Read the model definition and answer for the solid it produces. Units are mm, in the model's axes. Face numbers are marked on the shaded views. A direction names the side the tool comes from. Round coordinates to 2 decimals unless told otherwise and drop trailing zeros. Write each loop counter-clockwise with the first axis right and the second up, starting at its lowest first coordinate (ties: lowest second). Pieces come first, ordered by that corner, then holes. Notation, with made-up numbers: (-25.5, 51) -> (31.5, 51) arc R20 cw to (31.5, 77) -> close; hole circle Ø8 at (53.5, -36.75). An arc over 180 degrees is marked (long way). Return JSON: item names as keys, results as strings.
from build123d import *

# Parameters (mm, degrees)
F2_R = 0.15


with BuildPart() as f1:
    # F0 (on Front) → F1 (revolve)
    with BuildSketch(Plane.XZ):
        Polygon((-2, 2.75), (-2, 1.5), (2, 1.5), (2, 2.75), (1.5, 2.75), (1.5, 3.75), (2, 3.75), (2, 5.75), (1, 5.75), (1, 5), (-2, 5), (-2, 3.75), (-1.5, 3.75), (-1.5, 2.75), align=None)
    revolve(axis=Axis((-2.919078, 0, 0), (-1, 0, 0)))

    # F2
    f2_edges = [f1.edges().sort_by_distance(p)[0] for p in [
        (-2, 0, -5),
        (2, 0, -5.75),
        (-2, 0, -1.5),
        (2, 0, -1.5),
    ]]
    fillet(f2_edges, radius=F2_R)


solid = f1.part
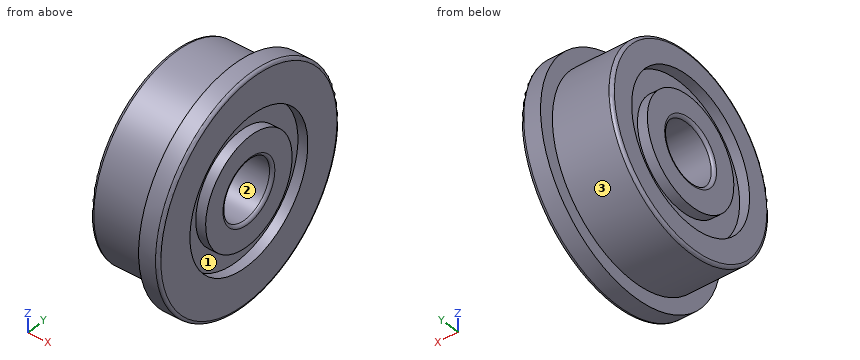
Item 1: Straight lines are drawn through the part: L1, parallel to Y at x = 1.85, z = 0; L2, parallel to Y at x = 1.85, z = 2.5; L3, parallel to X at y = 0.5, z = 2.75. For each, find the intervals that lie inside material, in ascending order. Write a range as [from, to].
Worked answers:
{"L1": "y = [-5.75, -3.75], [-2.75, -1.5], [1.5, 2.75], [3.75, 5.75]", "L2": "y = [-5.18, -2.8], [-1.15, 1.15], [2.8, 5.18]", "L3": "x = [-1.5, 1.5]"}
Item 2: A tool of negligible diameter and unlimited length cuts with its end or side. For the marked faces 1, 2 and 3, from which of +Z, -Z, +X, -X, +Y, -Y can it reach the whole face along a straight path? Write none if from no direction.
Worked answers:
{"face 1": "+X", "face 2": "+X, -X", "face 3": "-X"}
Item 3: Flat-ended cylindrical pins translate along their axes: pin 1 (2 mm diameter, centred on x = -0.5, z = 3, fed in from -Y); pin 2 (2 mm diameter, centred on x = -1.5, z = 0, fed in from +Y). Find the tip coordinate at first contact, or state that the pin passes through.
Worked answers:
{"pin 1": "stops at y = -4.58", "pin 2": "stops at y = 5"}
Item 4: Section A-A (x = 0.2) is taken. Give the vertices of the cut face in (y, z).
Worked answers:
{"outline": "circle Ø10 at (0, 0); hole circle Ø3 at (0, 0)"}
